Geometry: final body of the model. Coordinates: model frame, mm. A direction names the side the tool comes from. Coordinates: 2 decimals unless noted, no trailing zeros. Write each loop counter-clockwise with the first axis right and the second up, starting at its lowest first coordinate (ties: lowest second). Pieces come first, ordered by that corner, then holes. Notation, with made-up numbers: M 21,-32 L 48,-32 A17 cw 48,-8 Z; hole C 72,20.25 d2. An arc over 180 degrees is marked long. Write item = value, one per line. Start each with the question number.
Item 1: Section C-C on z = -9. Output: boundary loops of the cut face in (x, y).
Item 2: Section B-B on x = -1. Output: boundary loops of the cut face in (y, z).
Item 3: First-contact query: pin 1 Ø12 at (x, z) = (-54.5, -100) entering from +Y. Flat tip, straight axial feed; report the tip coordinate or a pass-through.
Item 4: Reachability of faces 1 (the flat face through (2, 0, 4)), 2 (the flat face through (-2, 19, -241.3)) from +Z, -Z, +X, -X, +Y, -Y: full face, straight path, thin tool, end or side. Return the list, or none.
Item 5: Ray query, L1, parallel to X at y = 23.25, z = -0.5; L2, parallel to Z at x = -24, y = 19; L3, parallel to Y at x = -89.5, z = 234. Return the intervals inside material, ascending. Write a range as [from, to].
Item 6: Section A-A on y = 19.25. Output: boundary loops of the cut face in (x, z), plus the area to 3 significant figures.
Item 7: Pull-direction query (X, two-part tool) for faces 3 (the flat face through (-127, 13, 4)), 4 (the flat face through (127, 13, -4)), 5 (the flat face through (2, 12.7, 3)), 6 (the flat face through (-2, 13, -254)); classes: +X half, -X half, draft (parallel to the pull), parting line (faces both ways), or undercut.
Autodesk Inventor part; units mm, degrees
ref_plane "YZ Plane" through (0, 0, 0) normal (1, 0, 0) x (0, 1, 0)
ref_plane "XZ Plane" through (0, 0, 0) normal (0, 1, 0) x (-1, 0, 0)
ref_plane "XY Plane" through (0, 0, 0) normal (0, 0, 1) x (1, 0, 0)
sketch "Sketch1" plane through (0, 0, 0) normal (0, 1, 0) x (-1, 0, 0)
  line L0 (-127, 254) -> (127, 254)
  line L1 (127, 254) -> (127, -254)
  line L2 (127, -254) -> (-127, -254)
  line L3 (-127, -254) -> (-127, 254)
  line L4 (-127, 254) -> (127, -254) construction
  line L5 (127, 254) -> (-127, -254) construction
  line L6 (-114.3, 241.3) -> (114.3, 241.3)
  line L7 (114.3, 241.3) -> (114.3, -241.3)
  line L8 (114.3, -241.3) -> (-114.3, -241.3)
  line L9 (-114.3, -241.3) -> (-114.3, 241.3)
  line L10 (-114.3, 241.3) -> (114.3, -241.3) construction
  line L11 (114.3, 241.3) -> (-114.3, -241.3) construction
  point P0 (0, 0)
  dimension "d0" = 508
  dimension "d1" = 254
  dimension "d2" = 482.6
  dimension "d3" = 228.6
extrude "Extrusion1" add sketch "Sketch1" along normal blind 12.7 contours L6 L7 L8 L9
extrude "Extrusion2" add sketch "Sketch1" along normal blind 25.4
properties part number "Potting Tray"
Responses:
q1.outline = M -127,0 L 127,0 L 127,25.4 L 114.3,25.4 L 114.3,12.7 L -114.3,12.7 L -114.3,25.4 L -127,25.4 Z
q2.outline = M 0,-254 L 25.4,-254 L 25.4,-241.3 L 12.7,-241.3 L 12.7,241.3 L 25.4,241.3 L 25.4,254 L 0,254 Z
q3.pin_1 = 12.7
q4.face_1 = +Z, -Z, +X, -X, -Y
q4.face_2 = +Y
q5.L1 = [-127, -114.3], [114.3, 127]
q5.L2 = [-254, -241.3], [241.3, 254]
q5.L3 = [0, 12.7]
q6.outline = M -127,-254 L 127,-254 L 127,254 L -127,254 Z; hole M -114.3,-241.3 L 114.3,-241.3 L 114.3,241.3 L -114.3,241.3 Z
q6.area = 18,700 mm²
q7.face_3 = -X half
q7.face_4 = +X half
q7.face_5 = undercut
q7.face_6 = draft
